```python
from build123d import *

# Parameters (mm, degrees)
ESQUISSE1_W        = 65.5
ESQUISSE1_H        = 41.5
BOSS_EXTRU_1_DEPTH = 5
COQUE1_T           = -3
CONG_1_R           = 5


with BuildPart() as part:
    # Esquisse1 → Boss.-Extru.1 (new body)
    with BuildSketch(Plane.XY):
        Rectangle(ESQUISSE1_W, ESQUISSE1_H)
    extrude(amount=BOSS_EXTRU_1_DEPTH)

    # Coque1
    coque1_openings = [part.faces().sort_by_distance(p)[0] for p in [
        (0, 0, 0),
    ]]
    offset(amount=COQUE1_T, openings=coque1_openings, kind=Kind.INTERSECTION)

    # Congé1
    cong_1_edges = [part.edges().sort_by_distance(p)[0] for p in [
        (29.75, -17.75, 1),
        (29.75, 17.75, 1),
        (-29.75, 17.75, 1),
        (-29.75, -17.75, 1),
        (32.75, -20.75, 2.5),
        (-32.75, -20.75, 2.5),
        (-32.75, 20.75, 2.5),
        (32.75, 20.75, 2.5),
    ]]
    fillet(cong_1_edges, radius=CONG_1_R)


solid = part.part
```
Design review of the part built by this model. Coordinates are the model's own, in mm. A direction names the side the tool comes from. Give positions to 0.01 mm unless a question says otherwise; leave off trailing zeros. Write each loop counter-clockwise with the first axis right and the second up, starting at its lowest first coordinate (ties: lowest second). Pieces come first, ordered by that corner, then holes. Notation, with made-up numbers: (40.5, 73) -> (49.5, 73) arc R25 cw to (49.5, 109) -> close; hole circle Ø10 at (87.5, 35). An arc over 180 degrees is marked (long way). Answer in a Markdown table with one row per item.
(1) Clearance check with a flat-ended pin moving along its axis: pin 1 (18 mm diameter, centred on x = 7, y = -3, fed in from -Z). State where the tip first meets the part, or that it passes through.
Results:
| item | result |
|---|---|
| pin 1 | z = 2 |
(2) For faces 1 (the flat face through (-32.75, 0, 2)), 2 (the flat face through (-29.75, 0, 1)), list the 3-axis set-ups (+Z, -Z, +X, -X, +Y, -Y) from which the entire face can be reached by the end or side of a thin tool; tool diameter is ignored.
Results:
| item | result |
|---|---|
| face 1 | +Z, -Z, -X, +Y, -Y |
| face 2 | -Z |
(3) Mouldability with a two-part tool opening along X and no side actions: class faces 3 (the cylindrical face through (28.32, 16.25, 0.99)), 4 (the cylindrical face through (-31.32, 19.25, 2.54)), 5 (the flat face through (-3, 19, 0)) as +X half, -X half, draft (parallel to the pull), parting line (faces both ways), or undercut.
Results:
| item | result |
|---|---|
| face 3 | undercut |
| face 4 | -X half |
| face 5 | draft |
(4) Consider section A-A (x = 28.5). State the section outline as (y, z) points.
Results:
| item | result |
|---|---|
| outline | (-20.69, 0) -> (-16.06, 0) -> (-16.06, 2) -> (16.06, 2) -> (16.06, 0) -> (20.69, 0) -> (20.69, 5) -> (-20.69, 5) -> close |
(5) To check wall thickness, follow probe 1 along X at (y, z) = (7, 0.8); probe 2 along Y at (x, z) = (12, 0.5); probe 3 along X at (y, z) = (-13, 1.3). State the ranges of each line that lie inside material, in increasing order.
Results:
| item | result |
|---|---|
| probe 1 | -32.75 to -29.75, 29.75 to 32.75 |
| probe 2 | -20.75 to -17.75, 17.75 to 20.75 |
| probe 3 | -32.75 to -29.74, 29.74 to 32.75 |
(6) Consider section B-B (y = -14.5). State the section outline as (x, z) points.
Results:
| item | result |
|---|---|
| outline | (-32.75, 0) -> (-29.43, 0) -> (-29.43, 2) -> (29.43, 2) -> (29.43, 0) -> (32.75, 0) -> (32.75, 5) -> (-32.75, 5) -> close |
